from build123d import *

# Parameters (mm, degrees)
SKETCH1_R           = 30
SKETCH1_R_2         = 1.5
BOSS_EXTRUDE1_DEPTH = 4
FILLET1_R           = 2


with BuildPart() as part:
    # Sketch1 → Boss-Extrude1 (new body)
    with BuildSketch(Plane(origin=(0, 0, 0), x_dir=(1, 0, 0), z_dir=(0, 1, 0))):
        with Locations(Location((0, 0, 0), (0, 0, 270))):
            Circle(SKETCH1_R)
        with Locations(Location((0, 23, 0), (0, 0, 270))):
            Circle(SKETCH1_R_2, mode=Mode.SUBTRACT)
        with Locations(Location((19.919084287, 11.500866025, 0), (0, 0, 270))):
            Circle(SKETCH1_R_2, mode=Mode.SUBTRACT)
        with Locations(Location((19.920084287, -11.499133975, 0), (0, 0, 270))):
            Circle(SKETCH1_R_2, mode=Mode.SUBTRACT)
        with Locations(Location((0.002, -23, 0), (0, 0, 270))):
            Circle(SKETCH1_R_2, mode=Mode.SUBTRACT)
        with Locations(Location((-19.917084287, -11.500866025, 0), (0, 0, 270))):
            Circle(SKETCH1_R_2, mode=Mode.SUBTRACT)
        with Locations(Location((-19.918084287, 11.499133975, 0), (0, 0, 270))):
            Circle(SKETCH1_R_2, mode=Mode.SUBTRACT)
    extrude(amount=BOSS_EXTRUDE1_DEPTH)

    # Fillet1
    fillet1_edges = [part.edges().sort_by_distance(p)[0] for p in [
        (0, 4, -30),
    ]]
    fillet(fillet1_edges, radius=FILLET1_R)


solid = part.part
Verification items for the finished model (mm, model axes). Round coordinates to 2 decimals unless told otherwise and drop trailing zeros. Use a Markdown table: item, result. Add a question column.
1. Section check A-A, the plane z = 11.5. Give the number of separate pieces and of enclosed holes in the cut face, plus the area to 3 significant figures.
2. Thickness scan on probe 1 along X at (y, z) = (3.35, 23); probe 2 along Z at (x, y) = (-19, 3); probe 3 along Z at (x, y) = (20, 0.9). Record the ranges inside material, lowest first. Write a range as [from, to].
3. Gauge pin test, flat ends, axial feed: pin 1 (2.5 mm diameter, centred on x = 19.92, z = -11.5, fed in from -Y) (3 decimals); pin 2 (1 mm diameter, centred on y = 0.5, z = 16, fed in from -X). Record the tip position at first contact, or that the pin passes through.
4. Release check for a two-part mould opening along X. For faces 1 (the face through (0, 0, 0)), 2 (the face through (0.07, 1.97, -24.5)), 3 (the face through (1.32, 0.99, -29.97)) record: released by +X, released by -X, zero draft, split by the parting line, or undercut.
Checks:
| question | item | result |
|---|---|---|
| 1 | separate pieces | 3 |
| 1 | enclosed holes | 0 |
| 1 | area | 196 mm^2 |
| 2 | probe 1 | x = [-18.43, -1.5], [1.5, 18.43] |
| 2 | probe 2 | z = [-22.87, -12.69], [-10.31, 10.31], [12.69, 22.87] |
| 2 | probe 3 | z = [-22.36, -13], [-10, 10], [13, 22.36] |
| 3 | pin 1 | passes through |
| 3 | pin 2 | stops at x = -25.69 |
| 4 | face 1 | zero draft |
| 4 | face 2 | undercut |
| 4 | face 3 | split by the parting line |
